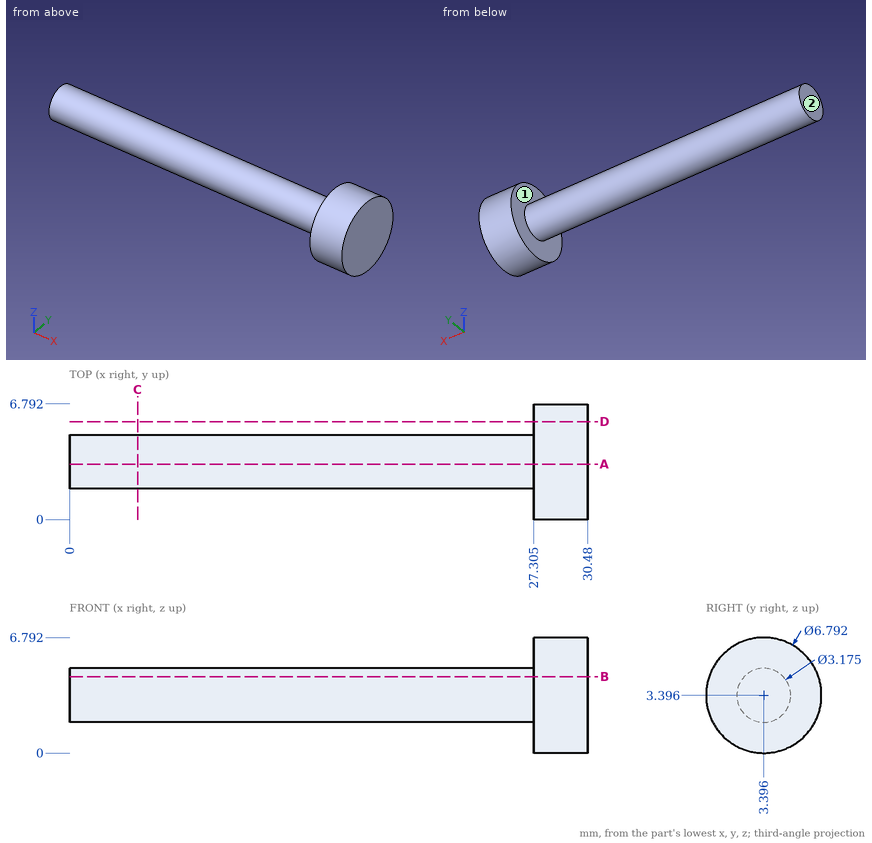
The drawing under review shows one solid part. Ordinate dimensions are in mm from its lowest x, y, z. A direction names the side the tool comes from. Give positions to 0.01 mm unless a question says otherwise; leave off trailing zeros. Loops run counter-clockwise (first coordinate to the right, second up) from the corner with the lowest first, then second, coordinate; pieces in that order, holes last. Notation, with made-up numbers: M 89,-21.5 L 120,-21.5 A28 ccw 120,9.5 Z; hole C -15.75,-26 d11. An arc over 180 degrees is marked long. One line per question, with ' | ' between items. Start each with the question number.
1. Add section B-B (z = 4.5). Write out the cut boundary in (x, y) (1 decimal).
2. Insertion check: P1, Ø3, axis at x = 10, z = 2.5, coming from the -Y side; P2, Ø1.5, axis at x = 22.5, y = 3, coming from the -Z side; P3, Ø3, axis at x = 22.5, y = 5.5, coming from the -Z side. Each pin has a flat end and moves straight along its axis. Give the tip position at first contact, or say it passes through.
3. To check wall thickness, follow L1, parallel to Z at x = 8.5, y = 3.25 (1 decimal); L2, parallel to Y at x = 8.5, z = 3.5; L3, parallel to X at y = 2.25, z = 6.5 (1 decimal). State the ranges of each line that lie inside material, in increasing order.
4. Add section D-D (y = 5.75). Write out the cut boundary in (x, z) (1 decimal).
5. For the marked faces 1 and 2, list the 3-axis set-ups (+Z, -Z, +X, -X, +Y, -Y) from which the entire face can be reached by the end or side of a thin tool; tool diameter is ignored.
6. Add section C-C (x = 4). Write out the cut boundary in (y, z) (1 decimal).
7. Add section A-A (y = 3.25). Write out the cut boundary in (x, z) (1 decimal), plus the area to 3 significant figures.
Worked out:
1) outline: M 0,2.3 L 27.3,2.3 L 27.3,0.2 L 30.5,0.2 L 30.5,6.6 L 27.3,6.6 L 27.3,4.5 L 0,4.5 Z
2) P1: stops at y = 1.81 | P2: stops at z = 1.81 | P3: stops at z = 1.93
3) L1: z = 1.8 to 5 | L2: y = 1.81 to 4.98 | L3: x = 27.3 to 30.5
4) outline: M 27.3,0.9 L 30.5,0.9 L 30.5,5.8 L 27.3,5.8 Z
5) face 1: -X | face 2: +Z, -Z, -X, +Y, -Y
6) outline: C 3.4,3.4 d3.2
7) outline: M 0,1.8 L 27.3,1.8 L 27.3,0 L 30.5,0 L 30.5,6.8 L 27.3,6.8 L 27.3,5 L 0,5 Z | area: 108 mm²
